Part model, mm, in its own coordinate system. Coordinates: 2 decimals unless noted, no trailing zeros. Write each loop counter-clockwise with the first axis right and the second up, starting at its lowest first coordinate (ties: lowest second). Pieces come first, ordered by that corner, then holes. Notation, with made-up numbers: (0, 24) - (43, 24) arc R16 ccw to (43, 39) - close; hole circle Ø7 at (-18.75, -0.75). An arc over 180 degrees is marked (long way). Use one line per item in the form item = value. Start each with the question number.
from build123d import *

# Parameters (mm, degrees)
SKETCH2_R           = 3.5
BOSS_EXTRUDE1_DEPTH = 1.016
FILLET1_R           = 12.7


with BuildPart() as part:
    # Sketch2 → Boss-Extrude1 (new body)
    with BuildSketch(Plane.XY):
        with BuildLine():
            Line((285.620600763, 115.53086565), (-273.179399237, 115.53086565))
            Line((-273.179399237, 115.53086565), (-273.179399237, -29.534072508))
            ThreePointArc((-273.179399237, -29.534072508), (-271.476904285, -35.885834684), (-266.825874397, -40.534629451))
            Line((-266.825874397, -40.534629451), (-111.025100537, -130.419691293))
            ThreePointArc((-111.025100537, -130.419691293), (-107.963661665, -131.686918852), (-104.678625377, -132.11913435))
            Line((-104.678625377, -132.11913435), (6.220600763, -132.11913435))
            Line((6.220600763, -132.11913435), (117.119826902, -132.11913435))
            ThreePointArc((117.119826902, -132.11913435), (120.40486319, -131.686918852), (123.466302062, -130.419691293))
            Line((123.466302062, -130.419691293), (279.267075922, -40.534629451))
            ThreePointArc((279.267075922, -40.534629451), (283.91810581, -35.885834684), (285.620600763, -29.534072508))
            Line((285.620600763, -29.534072508), (285.620600763, 115.53086565))
        make_face()
        with Locations((-209.679399237, 90.13086565)):
            Circle(SKETCH2_R, mode=Mode.SUBTRACT)
        with Locations((-101.729399237, 90.13086565)):
            Circle(SKETCH2_R, mode=Mode.SUBTRACT)
        with Locations((6.220600763, 90.13086565)):
            Circle(SKETCH2_R, mode=Mode.SUBTRACT)
        with Locations((114.170600763, 90.13086565)):
            Circle(SKETCH2_R, mode=Mode.SUBTRACT)
        with Locations((222.120600763, 90.13086565)):
            Circle(SKETCH2_R, mode=Mode.SUBTRACT)
    extrude(amount=BOSS_EXTRUDE1_DEPTH)

    # Fillet1
    fillet1_edges = [part.edges().sort_by_distance(p)[0] for p in [
        (-273.179399237, 115.53086565, 0.508),
        (285.620600763, 115.53086565, 0.508),
    ]]
    fillet(fillet1_edges, radius=FILLET1_R)


solid = part.part
Q1. Drill centre lines: probe 1 along Y at (x, z) = (-181.5, 0.1); probe 2 along X at (y, z) = (-89, 0.5); probe 3 along X at (y, z) = (-96, 0.75). Where is each one in solid material? Low to high.
Q2. Slice it at A-A (z = 0.4). List the corners of the cut face in (x, y), plus the area to 3 significant figures.
Q3. Pin check, flat tip, straight feed: P1, Ø11, axis at x = 114.17, y = 90.13, coming from the -Z side. Stop position of the tip, or through.
Q4. Slice it at B-B (x = 232.5). List the corners of the cut face in (y, z), plus the area to 3 significant figures.
Q5. Slice it at C-C (y = -115). List the corners of the cut face in (x, z), plus the area to 3 significant figures.
Solution:
q1.probe_1 = -89.76 to 115.53
q1.probe_2 = -182.82 to 195.26
q1.probe_3 = -170.69 to 183.13
q2.outline = (-273.18, -29.53) arc R12.7 ccw to (-266.83, -40.53) - (-111.03, -130.42) arc R12.7 ccw to (-104.68, -132.12) - (117.12, -132.12) arc R12.7 ccw to (123.47, -130.42) - (279.27, -40.53) arc R12.7 ccw to (285.62, -29.53) - (285.62, 102.83) arc R12.7 ccw to (272.92, 115.53) - (-260.48, 115.53) arc R12.7 ccw to (-273.18, 102.83) - close; hole circle Ø7 at (-209.68, 90.13); hole circle Ø7 at (-101.73, 90.13); hole circle Ø7 at (6.22, 90.13); hole circle Ø7 at (114.17, 90.13); hole circle Ø7 at (222.12, 90.13)
q2.area = 122,000 mm2
q3.P1 = 0
q4.outline = (-67.52, 0) - (115.53, 0) - (115.53, 1.02) - (-67.52, 1.02) - close
q4.area = 186 mm2
q5.outline = (-137.75, 0) - (150.19, 0) - (150.19, 1.02) - (-137.75, 1.02) - close
q5.area = 293 mm2
